from build123d import *

# Parameters (mm, degrees)
SKETCH_1_W               = 80
SKETCH_1_H               = 80
SKETCH_1_R               = 13.5
EXTRUDE_1_DEPTH          = 5
SKETCH_2_R               = 2.1
CUT_EXTRUDE_1_DEPTH      = 5
SKETCH_3_W               = 80
SKETCH_3_H               = 20
EXTRUDE_2_DEPTH          = 5
CUT_EXTRUDE_2_DEPTH      = 5
FILLET_1_R               = 1.5
FILLET_1_OF_MIRROR_1_R   = 1.5
EXTRUDE_3_DEPTH          = 3
FILLET_2_R               = 1.5
FILLET_2_OF_MIRROR_2_R   = 1.5
CUT_EXTRUDE_3_DEPTH      = 10
FILLET_3_R               = 3
CUT_EXTRUDE_4_DEPTH      = 10
CUT_EXTRUDE_4_DEPTH_BACK = 10


with BuildPart() as part:
    # 草图1 → 凸台-拉伸1 (new body)
    with BuildSketch(Plane.XY):
        Rectangle(SKETCH_1_W, SKETCH_1_H)
        Circle(SKETCH_1_R, mode=Mode.SUBTRACT)
    extrude(amount=EXTRUDE_1_DEPTH)

    # 草图2 → 切除-拉伸1 (cut)
    with BuildSketch(Plane.XY.offset(5)):
        with Locations((-12.374368671, 12.374368671)):
            Circle(SKETCH_2_R)
        with Locations((12.374368671, 12.374368671)):
            Circle(SKETCH_2_R)
        with Locations((-12.374368671, -12.374368671)):
            Circle(SKETCH_2_R)
        with Locations((12.374368671, -12.374368671)):
            Circle(SKETCH_2_R)
    extrude(amount=-CUT_EXTRUDE_1_DEPTH, mode=Mode.SUBTRACT)

    # 草图3 → 凸台-拉伸2 (add)
    with BuildSketch(Plane(origin=(0, 40, 0), x_dir=(1, 0, 0), z_dir=(0, 1, 0))):
        with Locations((0, -15)):
            Rectangle(SKETCH_3_W, SKETCH_3_H)
    extrude_2 = extrude(amount=-EXTRUDE_2_DEPTH)

    # 草图4 → 切除-拉伸2 (cut)
    with BuildSketch(Plane(origin=(0, 40, 0), x_dir=(1, 0, 0), z_dir=(0, 1, 0))):
        with BuildLine():
            Line((-31, -12.9), (-29, -12.9))
            ThreePointArc((-29, -12.9), (-26.9, -15), (-29, -17.1))
            Line((-29, -17.1), (-31, -17.1))
            ThreePointArc((-31, -17.1), (-33.1, -15), (-31, -12.9))
        make_face()
        with BuildLine():
            Line((-1, -12.9), (1, -12.9))
            ThreePointArc((1, -12.9), (3.1, -15), (1, -17.1))
            Line((1, -17.1), (-1, -17.1))
            ThreePointArc((-1, -17.1), (-3.1, -15), (-1, -12.9))
        make_face()
        with BuildLine():
            Line((29, -12.9), (31, -12.9))
            ThreePointArc((31, -12.9), (33.1, -15), (31, -17.1))
            Line((31, -17.1), (29, -17.1))
            ThreePointArc((29, -17.1), (26.9, -15), (29, -12.9))
        make_face()
    cut_extrude_2 = extrude(amount=-CUT_EXTRUDE_2_DEPTH, mode=Mode.SUBTRACT)

    # 圆角1
    fillet_1_edges = [part.edges().sort_by_distance(p)[0] for p in [
        (0, 35, 5),
    ]]
    fillet(fillet_1_edges, radius=FILLET_1_R)

    # 镜向1: 凸台-拉伸2, 切除-拉伸2 across plane
    add(extrude_2.mirror(Plane.ZX))
    add(cut_extrude_2.mirror(Plane.ZX), mode=Mode.SUBTRACT)

    # 圆角1 of 镜向1
    fillet_1_of_mirror_1_edges = [part.edges().sort_by_distance(p)[0] for p in [
        (0, -35, 5),
    ]]
    fillet(fillet_1_of_mirror_1_edges, radius=FILLET_1_OF_MIRROR_1_R)

    # 草图5 → 凸台-拉伸3 (add)
    with BuildSketch(Plane.ZY.offset(20)):
        Polygon((20, 35), (5, 5), (5, 35), align=None)
        Polygon((20, -35), (5, -5), (5, -35), align=None)
    extrude_3 = extrude(amount=EXTRUDE_3_DEPTH)

    # 圆角2
    fillet_2_edges = [part.edges().sort_by_distance(p)[0] for p in [
        (-20, 34.560660172, 5.439339828),
        (-23, 34.560660172, 5.439339828),
        (-20, 35, 13.25),
        (-21.5, 35, 20),
        (-23, 19.25, 5),
        (-23, 35, 13.25),
        (-20, 19.25, 5),
        (-21.5, 5, 5),
        (-20, -34.560660172, 5.439339828),
        (-23, -34.560660172, 5.439339828),
        (-20, -19.25, 5),
        (-21.5, -5, 5),
        (-23, -19.25, 5),
        (-23, -35, 13.25),
        (-20, -35, 13.25),
        (-21.5, -35, 20),
    ]]
    fillet(fillet_2_edges, radius=FILLET_2_R)

    # 镜向2: 凸台-拉伸3 across plane
    add(extrude_3.mirror(Plane(origin=(0, 0, 0), x_dir=(0, 0, 1), z_dir=(1, 0, 0))))

    # 圆角2 of 镜向2
    fillet_2_of_mirror_2_edges = [part.edges().sort_by_distance(p)[0] for p in [
        (20, 34.560660172, 5.439339828),
        (23, 34.560660172, 5.439339828),
        (20, 35, 13.25),
        (21.5, 35, 20),
        (23, 19.25, 5),
        (23, 35, 13.25),
        (20, 19.25, 5),
        (21.5, 5, 5),
        (20, -34.560660172, 5.439339828),
        (23, -34.560660172, 5.439339828),
        (20, -19.25, 5),
        (21.5, -5, 5),
        (23, -19.25, 5),
        (23, -35, 13.25),
        (20, -35, 13.25),
        (21.5, -35, 20),
    ]]
    fillet(fillet_2_of_mirror_2_edges, radius=FILLET_2_OF_MIRROR_2_R)

    # 草图6 → 切除-拉伸3 (cut)
    with BuildSketch(Plane.XY.offset(5)):
        with BuildLine():
            Line((-40, 30.5), (-28.878679656, 19.378679656))
            ThreePointArc((-28.878679656, 19.378679656), (-28.228361402, 18.40540961), (-28, 17.257359313))
            Line((-28, 17.257359313), (-28, -17.257359313))
            ThreePointArc((-28, -17.257359313), (-28.228361402, -18.40540961), (-28.878679656, -19.378679656))
            Line((-28.878679656, -19.378679656), (-40, -30.5))
            Line((-40, -30.5), (-40, 30.5))
        make_face()
        with BuildLine():
            Line((40, -30.5), (40, 30.5))
            Line((40, 30.5), (28.878679656, 19.378679656))
            ThreePointArc((28.878679656, 19.378679656), (28.228361402, 18.40540961), (28, 17.257359313))
            Line((28, 17.257359313), (28, -17.257359313))
            ThreePointArc((28, -17.257359313), (28.228361402, -18.40540961), (28.878679656, -19.378679656))
            Line((28.878679656, -19.378679656), (40, -30.5))
        make_face()
    extrude(amount=-CUT_EXTRUDE_3_DEPTH, mode=Mode.SUBTRACT)

    # 圆角3
    fillet_3_edges = [part.edges().sort_by_distance(p)[0] for p in [
        (-40, -30.5, 2.5),
        (-40, 30.5, 2.5),
        (40, 30.5, 2.5),
        (40, -30.5, 2.5),
    ]]
    fillet(fillet_3_edges, radius=FILLET_3_R)

    # 草图7 → 切除-拉伸4 (cut, two sides: drawn at the far end of the back side and taken through both)
    with BuildSketch(Plane.XY.offset(5).offset(-CUT_EXTRUDE_4_DEPTH_BACK)):
        with BuildLine():
            Line((-10, 35), (10, 35))
            ThreePointArc((10, 35), (18, 27), (10, 19))
            Line((10, 19), (-10, 19))
            ThreePointArc((-10, 19), (-18, 27), (-10, 35))
        make_face()
        with BuildLine():
            Line((-10, -19), (10, -19))
            ThreePointArc((10, -19), (18, -27), (10, -35))
            Line((10, -35), (-10, -35))
            ThreePointArc((-10, -35), (-18, -27), (-10, -19))
        make_face()
    extrude(amount=CUT_EXTRUDE_4_DEPTH + CUT_EXTRUDE_4_DEPTH_BACK, mode=Mode.SUBTRACT)


solid = part.part
Could you check a few things on this model? Use its own coordinates, in mm. A direction names the side the tool comes from. Give positions to 0.01 mm unless a question says otherwise; leave off trailing zeros. Order: outer loops, then holes, each group sorted by start corner. A loop starts at its lowest first (then second) coordinate and runs counter-clockwise, first axis right, second up.
Item 1: If we section it at A-A, the plane y = 27: Write out the boundary of the cut face in (x, z), plus the area to 3 significant figures.
Item 2: If we mould it in two halves opening along Y, with no side actions, what happens to faces 4 (the face through (23, 27, 10)), 5 (the face through (30, 38, 17.1)), 6 (the face through (-1, 40, 12))? For each: pulls with the +Y half, pulls with the -Y half, needs draft (parallel to the pull), parting line crosses it, or undercut.
Item 3: If we section it at C-C, the plane x = 2: Write out the boundary of the cut face in (y, z).
Item 4: I'm going to push flat-ended pins straight in: pin 1 (6.5 mm diameter, centred on y = -18, z = 13, fed in from -X); pin 2 (5.5 mm diameter, centred on y = 8, z = 1.5, fed in from -X); pin 3 (6.5 mm diameter, centred on y = 23.5, z = 12.5, fed in from +X). Where does each tip first touch, or does it pass through?
Item 5: If we section it at D-D, the plane z = 1.5: Count the separate pieces of the cut face and the enclosed holes in it, plus the area to 3 significant figures.
Item 6: I need wall thicknesses on line 1 (Y direction, x = 0, z = 2.15); line 2 (Y direction, x = 7.5, z = 9.5); line 3 (X direction, y = -31.5, z = 17). Which ranges of each line are inside material? Lowest first, please.
Item 7: For faces 1 (the face through (26.9, 37.5, 15)), 2 (the face through (-28.235, 18.421, 2.535)), 3 (the face through (-23, 27, 10)), which set-ups out of +Z, -Z, +X, -X, +Y, -Y let a thin tool reach every point of the face, with its end or its side?
Item 8: If we section it at B-B, the plane z = 22.5: Write out the boundary of the cut face in (x, y).
Values:
1. outline: (-36.5, 0) - (-18, 0) - (-18, 5) - (-18.5, 5) arc R1.5 cw to (-20, 6.5) - (-20, 16) - (-23, 16) - (-23, 6.5) arc R1.5 cw to (-24.5, 5) - (-36.5, 5) - close; (18, 0) - (36.5, 0) - (36.5, 5) - (24.5, 5) arc R1.5 cw to (23, 6.5) - (23, 16) - (20, 16) - (20, 6.5) arc R1.5 cw to (18.5, 5) - (18, 5) - close
1. area: 253 mm2
2. face 4: undercut
2. face 5: needs draft
2. face 6: pulls with the +Y half
3. outline: (-40, 0) - (-35, 0) - (-35, 13.15) - (-40, 13.15) - close; (-40, 16.85) - (-35, 16.85) - (-35, 25) - (-40, 25) - close; (-19, 0) - (-13.35, 0) - (-13.35, 5) - (-19, 5) - close; (13.35, 0) - (19, 0) - (19, 5) - (13.35, 5) - close; (35, 0) - (40, 0) - (40, 13.15) - (35, 13.15) - close; (35, 16.85) - (40, 16.85) - (40, 25) - (35, 25) - close
4. pin 1: stops at x = -23
4. pin 2: stops at x = -28
4. pin 3: stops at x = 23
5. separate pieces: 1
5. enclosed holes: 7
5. area: 3,550 mm2
6. line 1: y = -40 to -35, -19 to -13.5, 13.5 to 19, 35 to 40
6. line 2: y = -40 to -35, 35 to 40
6. line 3: x = -23 to -20, 20 to 23
7. face 1: +Y, -Y
7. face 2: +Z, -Z, -X
7. face 3: +Z, -X
8. outline: (-40, -40) - (40, -40) - (40, -35) - (-40, -35) - close; (-40, 35) - (40, 35) - (40, 40) - (-40, 40) - close
